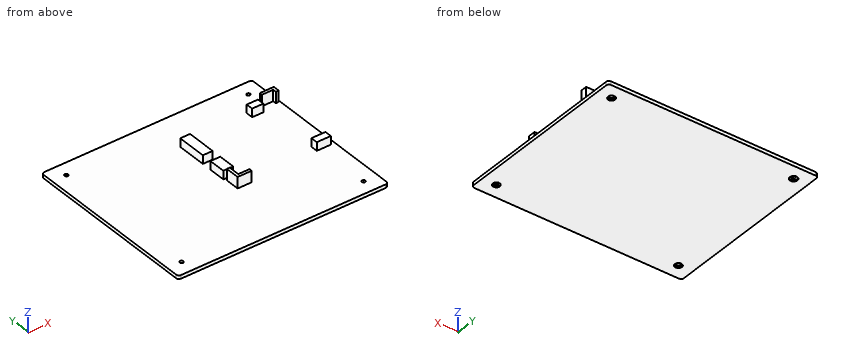
```python
from build123d import *

# Parameters (mm, degrees)
F0_W      = 150
F0_H      = 127.279
F1_DEPTH  = 2.5
F2_R      = 2.5
F2_R_2    = 2.718932
F2_R_3    = 2.518659
F3_DEPTH  = 1
F4_R      = 1.25
F5_DEPTH  = 1.501
F6_R      = 2
F8_DEPTH  = 8
F9_W      = 7
F9_H      = 12
F9_H_2    = 21
F9_W_2    = 8
F9_H_3    = 5
F10_DEPTH = 6
F11_W     = 10
F11_H     = 5
F12_DEPTH = 6


with BuildPart() as f1:
    # F0 (on Top) → F1 (new body)
    with BuildSketch(Plane.XY):
        with Locations((75, 63.6395)):
            Rectangle(F0_W, F0_H)
    extrude(amount=F1_DEPTH)

    # F2 (on face) → F3 (cut)
    with BuildSketch(Plane(origin=(0, 0, 0), x_dir=(1, 0, 0), z_dir=(0, 0, -1))):
        with Locations((10, -10)):
            Circle(F2_R)
        with Locations((140, -10)):
            Circle(F2_R)
        with Locations((10, -117.279)):
            Circle(F2_R_2)
        with Locations((140, -117.279)):
            Circle(F2_R_3)
    extrude(amount=-F3_DEPTH, mode=Mode.SUBTRACT)

    # F4 (on face) → F5 (cut, through all)
    with BuildSketch(Plane(origin=(0, 0, 1), x_dir=(1, 0, 0), z_dir=(0, 0, -1))):
        with Locations((10, -10)):
            Circle(F4_R)
        with Locations((10, -117.279)):
            Circle(F4_R)
        with Locations((140, -117.279)):
            Circle(F4_R)
        with Locations((140, -10)):
            Circle(F4_R)
    extrude(amount=-F5_DEPTH, mode=Mode.SUBTRACT)

    # F6
    f6_edges = [f1.edges().sort_by_distance(p)[0] for p in [
        (150, 0, 1.25),
        (0, 0, 1.25),
        (150, 127.279, 1.25),
        (0, 127.279, 1.25),
    ]]
    fillet(f6_edges, radius=F6_R)

    # F7 (on face) → F8 (join)
    with BuildSketch(Plane.XY.offset(2.5)):
        Polygon((89.045, 49.829), (81.045, 49.829), (81.045, 57.829), (79.045, 57.829), (79.045, 47.829), (89.045, 47.829), align=None)
        Polygon((139.095, 103.454), (147.095, 103.454), (147.095, 100.954), (149.095, 100.954), (149.095, 105.454), (139.095, 105.454), align=None)
    extrude(amount=F8_DEPTH)

    # F9 (on face) → F10 (join)
    with BuildSketch(Plane.XY.offset(2.5)):
        with Locations((81.545, 65.829)):
            Rectangle(F9_W, F9_H)
        with Locations((81.545, 89.454)):
            Rectangle(F9_W, F9_H_2)
        with Locations((132.045, 100.779)):
            Rectangle(F9_W_2, F9_H_3)
    extrude(amount=F10_DEPTH)

    # F11 (on face) → F12 (join)
    with BuildSketch(Plane.XY.offset(2.5)):
        with Locations((142.095, 52.329)):
            Rectangle(F11_W, F11_H)
    extrude(amount=F12_DEPTH)


solid = f1.part
```
Part model, mm, in its own coordinate system. Round coordinates to 2 decimals unless told otherwise and drop trailing zeros. Write each loop counter-clockwise with the first axis right and the second up, starting at its lowest first coordinate (ties: lowest second). Pieces come first, ordered by that corner, then holes. Notation, with made-up numbers: (-30, 12.5) -> (-7, 12.5) arc R21 cw to (-7, 18.5) -> close; hole circle Ø4 at (72.5, 24.25). An arc over 180 degrees is marked (long way). Return JSON: item names as keys, results as strings. Group by question number.
Q1. Pin check, flat tips, straight feed: pin 1 (1.8 mm diameter, centred on x = 80.5, z = 4, fed in from +Y); pin 2 (0.6 mm diameter, centred on y = 105, z = 6.5, fed in from -X) (3 decimals); pin 3 (3.5 mm diameter, centred on y = 103.5, z = 8, fed in from +X) (3 decimals). Stop position of each tip, or through.
Q2. Saw through at C-C on x = 115. Write the cut outline in (y, z), plus the area to 3 significant figures.
Q3. Saw through at A-A on z = 6.5. Write the cut outline in (x, y) (3 decimals).
Q4. Probe L1, parallel to Y at x = 10, z = 0.6; L2, parallel to X at y = 10, z = 0.75; L3, parallel to X at y = 10, z = 1.9. List the from-to ranges inside material, lowest first. Write a range as [from, to].
Q5. Saw through at B-B on y = 96.5. Write the cut outline in (x, z) (3 decimals).
Q6. Saw through at D-D on y = 77. Write the cut outline in (x, z), plus the area to 3 significant figures.
Answer:
{
 "1": {"pin 1": "y = 99.95", "pin 2": "x = 139.095", "pin 3": "x = 149.095"},
 "2": {"outline": "(0, 0) -> (127.28, 0) -> (127.28, 2.5) -> (0, 2.5) -> close", "area": "318 mm2"},
 "3": {"outline": "(78.045, 59.829) -> (85.045, 59.829) -> (85.045, 71.829) -> (78.045, 71.829) -> close; (78.045, 78.954) -> (85.045, 78.954) -> (85.045, 99.954) -> (78.045, 99.954) -> close; (79.045, 47.829) -> (89.045, 47.829) -> (89.045, 49.829) -> (81.045, 49.829) -> (81.045, 57.829) -> (79.045, 57.829) -> close; (128.045, 98.279) -> (136.045, 98.279) -> (136.045, 103.279) -> (128.045, 103.279) -> close; (137.095, 49.829) -> (147.095, 49.829) -> (147.095, 54.829) -> (137.095, 54.829) -> close; (139.095, 103.454) -> (147.095, 103.454) -> (147.095, 100.954) -> (149.095, 100.954) -> (149.095, 105.454) -> (139.095, 105.454) -> close"},
 "4": {"L1": "[0, 7.5], [12.5, 114.56], [120, 127.28]", "L2": "[0, 7.5], [12.5, 137.5], [142.5, 150]", "L3": "[0, 8.75], [11.25, 138.75], [141.25, 150]"},
 "5": {"outline": "(0, 0) -> (150, 0) -> (150, 2.5) -> (85.045, 2.5) -> (85.045, 8.5) -> (78.045, 8.5) -> (78.045, 2.5) -> (0, 2.5) -> close"},
 "6": {"outline": "(0, 0) -> (150, 0) -> (150, 2.5) -> (0, 2.5) -> close", "area": "375 mm2"}
}
